```python
from build123d import *

# Parameters (mm, degrees)
SKETCH1_R           = 101.6
BOSS_EXTRUDE1_DEPTH = 50.8
SKETCH2_R           = 76.2
BOSS_EXTRUDE2_DEPTH = 50.8
SKETCH3_R           = 12.7
CUT_EXTRUDE1_DEPTH  = 176.976362049
SKETCH4_R           = 25.4
BOSS_EXTRUDE3_DEPTH = 76.2


with BuildPart() as part:
    # Sketch1 → Boss-Extrude1 (new body)
    with BuildSketch(Plane(origin=(0, 0, 0), x_dir=(1, 0, 0), z_dir=(0, 1, 0))):
        with Locations(Location((0, 0, 0), (0, 0, 270))):
            Circle(SKETCH1_R)
    extrude(amount=BOSS_EXTRUDE1_DEPTH)

    # Sketch2 → Boss-Extrude2 (add)
    with BuildSketch(Plane(origin=(0, 50.8, 0), x_dir=(1, 0, 0), z_dir=(0, 1, 0))):
        with Locations(Location((0, 0, 0), (0, 0, 270))):
            Circle(SKETCH2_R)
    extrude(amount=BOSS_EXTRUDE2_DEPTH)

    # Sketch3 → Cut-Extrude1 (cut, through all)
    with BuildSketch(Plane(origin=(0, 101.6, 0), x_dir=(1, 0, 0), z_dir=(0, 1, 0))):
        with Locations(Location((0, 55.372, 0), (0, 0, 270))):
            Circle(SKETCH3_R)
        with Locations(Location((-55.372, 0, 0), (0, 0, 270))):
            Circle(SKETCH3_R)
        with Locations(Location((0, -55.372, 0), (0, 0, 270))):
            Circle(SKETCH3_R)
        with Locations(Location((55.372, 0, 0), (0, 0, 270))):
            Circle(SKETCH3_R)
    extrude(amount=-CUT_EXTRUDE1_DEPTH, mode=Mode.SUBTRACT)

    # Sketch4 → Boss-Extrude3 (add)
    with BuildSketch(Plane.XZ):
        with Locations(Location((0, 0, 0), (0, 0, 90))):
            Circle(SKETCH4_R)
    extrude(amount=BOSS_EXTRUDE3_DEPTH)


solid = part.part
```
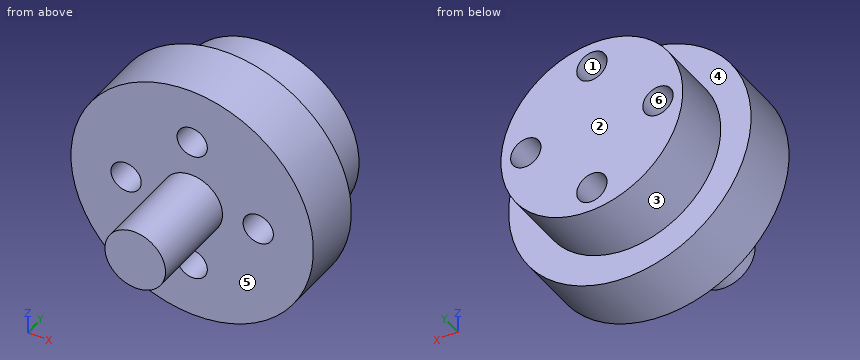
Geometry: final body of the model. Coordinates: model frame, mm. Face numbers are marked on the shaded views. A direction names the side the tool comes from. Round coordinates to 2 decimals unless told otherwise and drop trailing zeros. Order: outer loops, then holes, each group sorted by start corner. A loop starts at its lowest first (then second) coordinate and runs counter-clockwise, first axis right, second up. Notation, with made-up numbers: (-25.75, -1.75) - (-0.75, -1.75) arc R29 cw to (-0.75, 33.25) - close; hole circle Ø7 at (-1, 46.5). An arc over 180 degrees is marked (long way). Use CSV: the item, a comma, the result in double quotes. Start each with the question number.
Q1. Section query D-D (z = -53). Return loops of the section in (x, y), and give its area (3 significant figures).
Q2. First-contact query: pin 1 (2 mm diameter, centred on x = -55.5, y = 25, fed in from -Z); pin 2 (1 mm diameter, centred on y = 25, z = -36.5, fed in from +X); pin 3 (2 mm diameter, centred on x = -50, y = 72.5, fed in from +Z); pin 4 (23 mm diameter, centred on x = -55.372, z = 0, fed in from -Y). Flat tips, straight axial feed; report the tip coordinate or a pass-through.
Q3. Section query C-C (x = 51.5). Return loops of the section in (y, z).
Q4. Access query for the marked faces 4, 5 and 6. Directions: +Z, -Z, +X, -X, +Y, -Y. A direction counts if a zero-diameter tool reaches every point of the face in a straight line with its end or side. Return the directions, or none.
Q5. Mould query, pull axis Z, two halves, no side actions, for the marked faces 1, 2 and 3. Classes: +Z half, -Z half, draft (parallel to the pull), parting line (faces both ways), or undercut.
Q6. Section query B-B (z = -5.5). Return loops of the section in (x, y).
Q7. Section query A-A (x = 0). Return loops of the section in (y, z), and give its area (3 significant figures).
Q8. Material intervals for line 1 along Z through (x, y) = (2.5, 87.5); line 2 along Y through (x, z) = (-2.5, -37.5); line 3 along X through (y, z) = (44, 64), sorted ascending. Write a range as from..to.
Result set:
1,outline,"(-86.68, 0) - (-12.48, 0) - (-12.48, 101.6) - (-54.75, 101.6) - (-54.75, 50.8) - (-86.68, 50.8) - close; (12.48, 0) - (86.68, 0) - (86.68, 50.8) - (54.75, 50.8) - (54.75, 101.6) - (12.48, 101.6) - close"
1,area,"11,800 mm2"
2,pin 1,"stops at z = -85.75"
2,pin 2,"stops at x = 95.01"
2,pin 3,"stops at z = 58.36"
2,pin 4,"passes through"
3,outline,"(0, -87.58) - (50.8, -87.58) - (50.8, -56.16) - (101.6, -56.16) - (101.6, -12.1) - (0, -12.1) - close; (0, 12.1) - (101.6, 12.1) - (101.6, 56.16) - (50.8, 56.16) - (50.8, 87.58) - (0, 87.58) - close"
4,face 4,"+Y"
4,face 5,"-Y"
4,face 6,"+Y, -Y"
5,face 1,"undercut"
5,face 2,"draft"
5,face 3,"parting line"
6,outline,"(-101.45, 0) - (-66.82, 0) - (-66.82, 101.6) - (-76, 101.6) - (-76, 50.8) - (-101.45, 50.8) - close; (-43.92, 0) - (-24.8, 0) - (-24.8, -76.2) - (24.8, -76.2) - (24.8, 0) - (43.92, 0) - (43.92, 101.6) - (-43.92, 101.6) - close; (66.82, 0) - (101.45, 0) - (101.45, 50.8) - (76, 50.8) - (76, 101.6) - (66.82, 101.6) - close"
7,outline,"(-76.2, -25.4) - (0, -25.4) - (0, -42.67) - (101.6, -42.67) - (101.6, 42.67) - (0, 42.67) - (0, 25.4) - (-76.2, 25.4) - close; (0, -101.6) - (50.8, -101.6) - (50.8, -76.2) - (101.6, -76.2) - (101.6, -68.07) - (0, -68.07) - close; (0, 68.07) - (101.6, 68.07) - (101.6, 76.2) - (50.8, 76.2) - (50.8, 101.6) - (0, 101.6) - close"
7,area,"16,800 mm2"
8,line 1,"z = -76.16..-67.82, -42.92..42.92, 67.82..76.16"
8,line 2,"y = 0..101.6"
8,line 3,"x = -78.91..-9.32, 9.32..78.91"
